```python
from build123d import *

# Parameters (mm, degrees)
F0_R     = 22.260195
F1_DEPTH = 25.4
F3_DEPTH = 7.366
F4_R     = 16.674385
F5_DEPTH = 25.401
F6_W     = 20.843665
F6_H     = 9.852567
F7_DEPTH = 17.272
F9_DEPTH = 26.967665


with BuildPart() as f1:
    # F0 (on Top) → F1 (new body)
    with BuildSketch(Plane.XY):
        Circle(F0_R)
    extrude(amount=F1_DEPTH)

    # F2 (on face) → F3 (join)
    with BuildSketch(Plane(origin=(0, 0, 0), x_dir=(1, 0, 0), z_dir=(0, 0, -1))):
        with BuildLine():
            ThreePointArc((22.260195, 0), (15.740335, -15.740335), (0, -22.260195))
            Line((0, -22.260195), (54.766204, -22.260195))
            Line((54.766204, -22.260195), (54.480962, 22.260195))
            Line((54.480962, 22.260195), (0, 22.260195))
            ThreePointArc((0, 22.260195), (15.740335, 15.740335), (22.260195, 0))
        make_face()
    extrude(amount=-F3_DEPTH)

    # F4 (on face) → F5 (cut, through all)
    with BuildSketch(Plane.XY.offset(25.4)):
        Circle(F4_R)
    extrude(amount=-F5_DEPTH, mode=Mode.SUBTRACT)

    # F6 (on face) → F7 (join)
    with BuildSketch(Plane.XY.offset(7.366)):
        with Locations((32.079024, 0.219813)):
            Rectangle(F6_W, F6_H)
    extrude(amount=F7_DEPTH)

    # F8 (on face) → F9 (cut, through all)
    with BuildSketch(Plane.XZ.offset(4.706471)):
        Polygon((42.500857, 24.638), (21.756962, 24.638), (42.500857, 7.366), align=None)
    extrude(amount=-F9_DEPTH, mode=Mode.SUBTRACT)


solid = f1.part
```
CAD build for the part. Positions are in the model's coordinates, mm. A direction names the side the tool comes from. Round coordinates to 2 decimals unless told otherwise and drop trailing zeros. Loops run counter-clockwise (first coordinate to the right, second up) from the corner with the lowest first, then second, coordinate; pieces in that order, holes last. Notation, with made-up numbers: (9.5, -4) - (34.5, -4) arc R22 cw to (34.5, 5) - close; hole circle Ø8 at (88, -27). An arc over 180 degrees is marked (long way). Return JSON: item names as keys, results as strings. Group by question number.
Q1. Band-saw the part on D-D on x = -6.5. Give the cut face in (y, z).
Q2. Drill centre lines: line 1 along Y through (x, z) = (0, 20.25); line 2 along X through (y, z) = (-1, 2); line 3 along Y through (x, z) = (14.5, 13.5). Where is each one in solid material? Low to high. Write a range as [from, to].
Q3. Band-saw the part on A-A on x = 11.5. Give the cut face in (y, z).
Q4. Band-saw the part on B-B on y = 0. Give the cut face in (x, z).
Q5. Flat gauge pins, fed straight in: pin 1 Ø8 at (y, z) = (-2.5, 10.5) entering from +X; pin 2 Ø5 at (x, z) = (33, 14) entering from -Y; pin 3 Ø5 at (x, z) = (10, 16) entering from +Y. Where does each tip first touch, or does it go through?
Q6. Band-saw the part on C-C on z = 4.75. Give the cut face in (x, y), plus the area to 3 significant figures.
Q7. Two-plate mould, pull along Y, no slides. Class faces 4 (the face through (30, 5.146, 14)), 5 (the face through (24, 0, 0)), 6 (the face through (-12.29, 11.27, 12.88)): +Y half, -Y half, draft (parallel to the pull), parting line (faces both ways), or undercut.
Q8. Tool access for faces 1 (the face through (-22.24, 0.98, 15.34)), 2 (the face through (30, -4.706, 14)), 3 (the face through (39, -5, 7.366)): list every direction of +Z, -Z, +X, -X, +Y, -Y with a clear straight run to the whole face (end or side of a thin tool).
Solutions:
{
 "1": {"outline": "(-21.29, 0) - (-15.36, 0) - (-15.36, 25.4) - (-21.29, 25.4) - close; (15.36, 0) - (21.29, 0) - (21.29, 25.4) - (15.36, 25.4) - close"},
 "2": {"line 1": "y = [-22.26, -16.67], [16.67, 22.26]", "line 2": "x = [-22.24, -16.64], [16.64, 54.62]", "line 3": "y = [-16.89, -8.23], [8.23, 16.89]"},
 "3": {"outline": "(-22.26, 0) - (-12.07, 0) - (-12.07, 25.4) - (-19.06, 25.4) - (-19.06, 7.37) - (-22.26, 7.37) - close; (12.07, 0) - (22.26, 0) - (22.26, 7.37) - (19.06, 7.37) - (19.06, 25.4) - (12.07, 25.4) - close"},
 "4": {"outline": "(-22.26, 0) - (-16.67, 0) - (-16.67, 25.4) - (-22.26, 25.4) - close; (16.67, 0) - (54.62, 0) - (54.62, 7.37) - (42.5, 7.37) - (21.76, 24.64) - (22.26, 24.64) - (22.26, 25.4) - (16.67, 25.4) - close"},
 "5": {"pin 1": "stops at x = 54.62", "pin 2": "stops at y = -4.71", "pin 3": "stops at y = 20.96"},
 "6": {"outline": "(0, -22.26) - (54.48, -22.26) - (54.77, 22.26) - (0, 22.26) arc R22.26 ccw to start; hole circle Ø33.35 at (0, 0)", "area": "2,340 mm^2"},
 "7": {"face 4": "+Y half", "face 5": "draft", "face 6": "undercut"},
 "8": {"face 1": "+Z", "face 2": "+Z, +X, -Y", "face 3": "+Z, +X"}
}
